Read the model definition and answer for the solid it produces. Units are mm, in the model's axes. A direction names the side the tool comes from. Coordinates: 2 decimals unless noted, no trailing zeros. Loops run counter-clockwise (first coordinate to the right, second up) from the corner with the lowest first, then second, coordinate; pieces in that order, holes last.
Q1. Straight lines are drawn through the part: line 1 (Y direction, x = -4.5, z = 3.5); line 2 (X direction, y = 1.75, z = 1.5); line 3 (X direction, y = 4.5, z = 5.75). For each, find the intervals that lie inside material, in ascending order.
Q2. Section D-D (x = -8.75) is taken. Give the vertices of the cut face in (y, z), then the cut area to 3 significant figures.
Q3. Section B-B (x = -2.25) is taken. Give the vertices of the cut face in (y, z).
Q4. Which of the six approach directions +Z, -Z, +X, -X, +Y, -Y give full straight-line access (tool end or side, diameter ignored) to faces 1 (the face through (8, 2, 3)), 2 (the face through (9, 0, 1)), 3 (the face through (1, 0, 5.5)), 4 (the face through (2.4, 3.2, 6))?
Q5. Section A-A (z = 4.25) is taken. Give the vertices of the cut face in (x, y), then the cut area to 3 significant figures.
Q6. Flat-ended cylindrical pins translate along their axes: P1, Ø1.5, axis at x = 8, z = 1.5, coming from the +Y side; P2, Ø2.5, axis at x = 8.5, z = 1, coming from the -Y side; P3, Ø1.5, axis at x = -8, y = 4, coming from the +Z side. Find the tip coordinate at first contact, or state that the pin passes through.
Q7. Section C-C (z = 1.75) is taken. Give the vertices of the cut face in (x, y).
from build123d import *

# Parameters (mm, degrees)
SKETCH1_W           = 13
SKETCH1_H           = 15.8
BOSS_EXTRUDE1_DEPTH = 6.5
SHELL1_T            = -1
CUT_EXTRUDE2_DEPTH  = 2.5
SKETCH3_W           = 5
SKETCH3_H           = 7
BOSS_EXTRUDE2_DEPTH = 3
SKETCH4_R           = 1.75
CUT_EXTRUDE3_DEPTH  = 5


with BuildPart() as part:
    # Sketch1 → Boss-Extrude1 (new body)
    with BuildSketch(Plane.XY):
        Rectangle(SKETCH1_W, SKETCH1_H)
    extrude(amount=BOSS_EXTRUDE1_DEPTH)

    # Shell1
    shell1_openings = [part.faces().sort_by_distance(p)[0] for p in [
        (0, 0, 0),
    ]]
    offset(amount=SHELL1_T, openings=shell1_openings, kind=Kind.INTERSECTION)

    # Sketch2 → Cut-Extrude2 (cut)
    with BuildSketch(Plane(origin=(0, 0, 5.5), x_dir=(-1, 0, 0), z_dir=(0, 0, -1))):
        with BuildLine():
            Line((-5.105072533, -5.71873747), (4.265069263, 6.036531329))
            ThreePointArc((4.265069263, 6.036531329), (4.865789922, 6.104354629), (4.933613222, 5.50363397))
            Line((4.933613222, 5.50363397), (-4.436528574, -6.251634828))
            ThreePointArc((-4.436528574, -6.251634828), (-5.037249233, -6.319458129), (-5.105072533, -5.71873747))
        make_face()
        with BuildLine():
            Line((-3.479803699, -5.763578957), (4.428264236, 4.157451726))
            ThreePointArc((4.428264236, 4.157451726), (4.923771659, 4.213396112), (4.979716045, 3.71788869))
            Line((4.979716045, 3.71788869), (-2.92835189, -6.203141993))
            ThreePointArc((-2.92835189, -6.203141993), (-3.423859312, -6.259086379), (-3.479803699, -5.763578957))
        make_face()
        with BuildLine():
            Line((-1.836206221, -5.738869047), (4.404824726, 2.090787959))
            ThreePointArc((4.404824726, 2.090787959), (4.949248544, 2.152255164), (5.01071575, 1.607831346))
            Line((5.01071575, 1.607831346), (-1.230315197, -6.22182566))
            ThreePointArc((-1.230315197, -6.22182566), (-1.774739016, -6.283292866), (-1.836206221, -5.738869047))
        make_face()
        with BuildLine():
            Line((0.230638955, -5.747393414), (4.533785605, -0.348900345))
            ThreePointArc((4.533785605, -0.348900345), (5.051093924, -0.290494567), (5.109499701, -0.807802886))
            Line((5.109499701, -0.807802886), (0.806353052, -6.206295955))
            ThreePointArc((0.806353052, -6.206295955), (0.289044733, -6.264701733), (0.230638955, -5.747393414))
        make_face()
        with BuildLine():
            Line((2.662525183, -5.734264805), (4.528368603, -3.393479423))
            ThreePointArc((4.528368603, -3.393479423), (5.065343895, -3.33285318), (5.125970138, -3.869828472))
            Line((5.125970138, -3.869828472), (3.260126717, -6.210613854))
            ThreePointArc((3.260126717, -6.210613854), (2.723151425, -6.271240097), (2.662525183, -5.734264805))
        make_face()
        with BuildLine():
            Line((-5.076600471, -3.401160753), (2.673836157, 5.986195062))
            ThreePointArc((2.673836157, 5.986195062), (3.1909607, 6.035588301), (3.24035394, 5.518463758))
            Line((3.24035394, 5.518463758), (-4.510082688, -3.868892057))
            ThreePointArc((-4.510082688, -3.868892057), (-5.027207231, -3.918285297), (-5.076600471, -3.401160753))
        make_face()
        with BuildLine():
            Line((-5.075895555, -1.176345618), (1.030282687, 6.219478717))
            ThreePointArc((1.030282687, 6.219478717), (1.546120318, 6.268749037), (1.595390638, 5.752911406))
            Line((1.595390638, 5.752911406), (-4.510787604, -1.642912929))
            ThreePointArc((-4.510787604, -1.642912929), (-5.026625235, -1.692183249), (-5.075895555, -1.176345618))
        make_face()
        with BuildLine():
            Line((-5.088414127, 1.144510192), (-0.889859337, 6.229814365))
            ThreePointArc((-0.889859337, 6.229814365), (-0.351167486, 6.281267609), (-0.299714242, 5.742575759))
            Line((-0.299714242, 5.742575759), (-4.498269031, 0.657271586))
            ThreePointArc((-4.498269031, 0.657271586), (-5.036960882, 0.605818341), (-5.088414127, 1.144510192))
        make_face()
        with BuildLine():
            Line((-5.129445403, 3.72103873), (-3.030168008, 6.263690816))
            ThreePointArc((-3.030168008, 6.263690816), (-2.416568429, 6.322298886), (-2.35796036, 5.708699307))
            Line((-2.35796036, 5.708699307), (-4.457237755, 3.166047221))
            ThreePointArc((-4.457237755, 3.166047221), (-5.070837334, 3.107439152), (-5.129445403, 3.72103873))
        make_face()
    extrude(amount=-CUT_EXTRUDE2_DEPTH, mode=Mode.SUBTRACT)

    # Sketch3 → Boss-Extrude2 (add)
    with BuildSketch(Plane(origin=(0, 0, 0), x_dir=(-1, 0, 0), z_dir=(0, 0, -1))):
        with Locations((9, 3.5)):
            Rectangle(SKETCH3_W, SKETCH3_H)
        with Locations((-9, 3.5)):
            Rectangle(SKETCH3_W, SKETCH3_H)
    extrude(amount=-BOSS_EXTRUDE2_DEPTH)

    # Sketch4 → Cut-Extrude3 (cut)
    with BuildSketch(Plane(origin=(0, 0, 0), x_dir=(-1, 0, 0), z_dir=(0, 0, -1))):
        with Locations((-9.18918569, 3.702089239)):
            Circle(SKETCH4_R)
        with Locations((9.130886442, 3.702089239)):
            Circle(SKETCH4_R)
    extrude(amount=-CUT_EXTRUDE3_DEPTH, mode=Mode.SUBTRACT)


solid = part.part
Numbers:
1. line 1: y = -7.9 to -6.9, 6.9 to 7.9
1. line 2: x = -11.5 to -5.5, 5.5 to 11.5
1. line 3: x = -6.5 to -4.13, -3.04 to -2.4, -1.45 to -0.56, 0.39 to 1.33, 2.32 to 3.36, 4.49 to 6.5
2. outline: (0, 0) - (1.99, 0) - (1.99, 3) - (0, 3) - close; (5.41, 0) - (7, 0) - (7, 3) - (5.41, 3) - close
2. area: 10.8 mm2
3. outline: (-7.9, 0) - (-6.9, 0) - (-6.9, 5.5) - (-4.4, 5.5) - (-4.4, 6.5) - (-7.9, 6.5) - close; (-3.21, 5.5) - (-1.86, 5.5) - (-1.86, 6.5) - (-3.21, 6.5) - close; (-0.61, 5.5) - (0.29, 5.5) - (0.29, 6.5) - (-0.61, 6.5) - close; (1.42, 5.5) - (2.14, 5.5) - (2.14, 6.5) - (1.42, 6.5) - close; (3.51, 5.5) - (4.32, 5.5) - (4.32, 6.5) - (3.51, 6.5) - close; (5.47, 5.5) - (6.9, 5.5) - (6.9, 0) - (7.9, 0) - (7.9, 6.5) - (5.47, 6.5) - close
4. face 1: +Z, +X, +Y, -Y
4. face 2: +Z, -Z, +X, -Y
4. face 3: -Z
4. face 4: +Z, -Z
5. outline: (-6.5, -7.9) - (6.5, -7.9) - (6.5, 7.9) - (-6.5, 7.9) - close; hole (-5.5, -6.9) - (5.5, -6.9) - (5.5, 6.9) - (-5.5, 6.9) - close
5. area: 53.6 mm2
6. P1: stops at y = 7
6. P2: stops at y = 0
6. P3: stops at z = 3
7. outline: (-11.5, 0) - (-6.5, 0) - (-6.5, -7.9) - (6.5, -7.9) - (6.5, 0) - (11.5, 0) - (11.5, 7) - (6.5, 7) - (6.5, 7.9) - (-6.5, 7.9) - (-6.5, 7) - (-11.5, 7) - close; hole circle Ø3.5 at (-9.13, 3.7); hole (-5.5, -6.9) - (5.5, -6.9) - (5.5, 6.9) - (-5.5, 6.9) - close; hole circle Ø3.5 at (9.19, 3.7)
